from build123d import *

# Parameters (mm, degrees)
SKETCH1_R           = 40
BOSS_EXTRUDE1_DEPTH = 13
SKETCH3_R           = 35
CUT_EXTRUDE1_DEPTH  = 10
SKETCH4_R           = 33
BOSS_EXTRUDE2_DEPTH = 4
SKETCH7_R           = 40
SKETCH7_R_2         = 35
BOSS_EXTRUDE3_DEPTH = 3
SKETCH8_R           = 35.5
CUT_EXTRUDE2_DEPTH  = 13
SKETCH9_R           = 33.75
BOSS_EXTRUDE6_DEPTH = 7
SKETCH10_R          = 28.645528411
CUT_EXTRUDE3_DEPTH  = 6
SKETCH11_R          = 33.75
SKETCH11_R_2        = 28.645528411
BOSS_EXTRUDE8_DEPTH = 3


with BuildPart() as part:
    # Sketch1 → Boss-Extrude1 (new body)
    with BuildSketch(Plane(origin=(0, 0, 0), x_dir=(1, 0, 0), z_dir=(0, 1, 0))):
        with Locations(Location((0, 0, 0), (0, 0, 270))):
            Circle(SKETCH1_R)
    extrude(amount=BOSS_EXTRUDE1_DEPTH)

    # Sketch3 → Cut-Extrude1 (cut)
    with BuildSketch(Plane(origin=(0, 13, 0), x_dir=(1, 0, 0), z_dir=(0, 1, 0))):
        with Locations(Location((0, 0, 0), (0, 0, 270))):
            Circle(SKETCH3_R)
    extrude(amount=-CUT_EXTRUDE1_DEPTH, mode=Mode.SUBTRACT)

    # Sketch4 → Boss-Extrude2 (add)
    with BuildSketch(Plane(origin=(0, 3, 0), x_dir=(1, 0, 0), z_dir=(0, 1, 0))):
        with Locations(Location((0, 0, 0), (0, 0, 270))):
            Circle(SKETCH4_R)
    extrude(amount=BOSS_EXTRUDE2_DEPTH)

    # Sketch7 → Boss-Extrude3 (add)
    with BuildSketch(Plane(origin=(0, 13, 0), x_dir=(1, 0, 0), z_dir=(0, 1, 0))):
        with Locations(Location((0, 0, 0), (0, 0, 270))):
            Circle(SKETCH7_R)
        with Locations(Location((0, 0, 0), (0, 0, 270))):
            Circle(SKETCH7_R_2, mode=Mode.SUBTRACT)
    extrude(amount=BOSS_EXTRUDE3_DEPTH)

    # Sketch8 → Cut-Extrude2 (cut)
    with BuildSketch(Plane(origin=(0, 16, 0), x_dir=(1, 0, 0), z_dir=(0, 1, 0))):
        with Locations(Location((0, 0, 0), (0, 0, 270))):
            Circle(SKETCH8_R)
    extrude(amount=-CUT_EXTRUDE2_DEPTH, mode=Mode.SUBTRACT)

    # Sketch9 → Boss-Extrude6 (add)
    with BuildSketch(Plane(origin=(0, 3, 0), x_dir=(1, 0, 0), z_dir=(0, 1, 0))):
        with Locations(Location((0, 0, 0), (0, 0, 90))):
            Circle(SKETCH9_R)
    extrude(amount=BOSS_EXTRUDE6_DEPTH)

    # Sketch10 → Cut-Extrude3 (cut)
    with BuildSketch(Plane(origin=(0, 10, 0), x_dir=(1, 0, 0), z_dir=(0, 1, 0))):
        with Locations(Location((0, 0, 0), (0, 0, 270))):
            Circle(SKETCH10_R)
    extrude(amount=-CUT_EXTRUDE3_DEPTH, mode=Mode.SUBTRACT)

    # Sketch11 → Boss-Extrude8 (add)
    with BuildSketch(Plane(origin=(0, 10, 0), x_dir=(1, 0, 0), z_dir=(0, 1, 0))):
        with Locations(Location((0, 0, 0), (0, 0, 90))):
            Circle(SKETCH11_R)
        with Locations(Location((0, 0, 0), (0, 0, 270))):
            Circle(SKETCH11_R_2, mode=Mode.SUBTRACT)
    extrude(amount=BOSS_EXTRUDE8_DEPTH)


solid = part.part
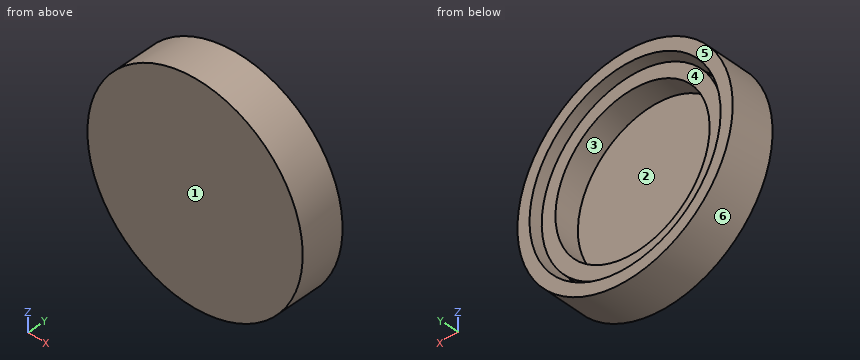
The listing builds one solid part. Answer for the finished solid, in the listing's coordinates (mm). Face numbers are marked on the shaded views. A direction names the side the tool comes from. Give positions to 0.01 mm unless a question says otherwise; leave off trailing zeros. Write each loop counter-clockwise with the first axis right and the second up, starting at its lowest first coordinate (ties: lowest second). Pieces come first, ordered by that corner, then holes.
Item 1: Determine the mould class of the marked faces 3, 4, 5 and 6 for opening direction Z: released by +Z, released by -Z, zero draft, split by the parting line, or undercut.
Item 2: Section D-D, the plane z = 30 is taken. Write down the section's boundary in (x, y), plus the area to 3 significant figures.
Item 3: Which of the six approach directions +Z, -Z, +X, -X, +Y, -Y give full straight-line access (tool end or side, diameter ignored) to the marked faces 1 and 2?
Item 4: Find the intervals of material crossed by line 1 along X through (y, z) = (11.75, 0); line 2 along Z through (x, y) = (-8.5, 3.5); line 3 along X through (y, z) = (3.25, 23.5), in increasing order.
Item 5: Section A-A, the plane y = 7.75 is taken. Write down the section's boundary in (x, z), plus the area to 3 significant figures.
Item 6: Section C-C, the plane x = 0 is taken. Write down the section's boundary in (y, z), plus the area to 3 significant figures.
Item 7: Flat-ended cylindrical pins translate along their axes: P1, Ø6, axis at y = 7.5, z = 31, coming from the -X side; P2, Ø21.5, axis at x = 10, z = -12.5, coming from the +Y side; P3, Ø1.5, axis at x = 20.5, z = 27, coming from the +Y side. Find the tip coordinate at first contact, or state that the pin passes through.
Item 8: Section B-B, the plane z = 0 is taken. Write down the section's boundary in (x, y), plus the area to 3 significant figures.
Completed:
1. face 3: undercut
1. face 4: undercut
1. face 5: zero draft
1. face 6: split by the parting line
2. outline: (-26.46, 0) - (26.46, 0) - (26.46, 16) - (18.98, 16) - (18.98, 3) - (15.46, 3) - (15.46, 13) - (-15.46, 13) - (-15.46, 3) - (-18.98, 3) - (-18.98, 16) - (-26.46, 16) - close
2. area: 662 mm2
3. face 1: +Z, -Z, +X, -X, -Y
3. face 2: +Y
4. line 1: x = -40 to -35.5, -33.75 to -28.65, 28.65 to 33.75, 35.5 to 40
4. line 2: z = -39.09 to -34.47, -32.66 to 32.66, 34.47 to 39.09
4. line 3: x = -32.37 to -26.61, -24.22 to 24.22, 26.61 to 32.37
5. outline: circle Ø80 at (0, 0); circle Ø67.5 at (0, 0); hole circle Ø71 at (0, 0); hole circle Ø57.29 at (0, 0)
5. area: 2,070 mm2
6. outline: (0, -40) - (16, -40) - (16, -35.5) - (3, -35.5) - (3, -33.75) - (13, -33.75) - (13, -28.65) - (4, -28.65) - (4, 28.65) - (13, 28.65) - (13, 33.75) - (3, 33.75) - (3, 35.5) - (16, 35.5) - (16, 40) - (0, 40) - close
6. area: 516 mm2
7. P1: stops at x = -28.57
7. P2: stops at y = 4
7. P3: stops at y = 13
8. outline: (-40, 0) - (40, 0) - (40, 16) - (35.5, 16) - (35.5, 3) - (33.75, 3) - (33.75, 13) - (28.65, 13) - (28.65, 4) - (-28.65, 4) - (-28.65, 13) - (-33.75, 13) - (-33.75, 3) - (-35.5, 3) - (-35.5, 16) - (-40, 16) - close
8. area: 516 mm2
